Check sheet for the modelled part. Datum: model origin and axes. Units: mm. A direction names the side the tool comes from. Coordinates: 2 decimals unless noted, no trailing zeros. Loops run counter-clockwise (first coordinate to the right, second up) from the corner with the lowest first, then second, coordinate; pieces in that order, holes last. Notation, with made-up numbers: M 7,6.5 L 25,6.5 A26 cw 25,34.5 Z; hole C -23.5,62 d2. An arc over 180 degrees is marked long. Return JSON: item names as keys, results as strings.
from build123d import *

# Parameters (mm, degrees)
P_IDAT_VYSUNUT_M1_DEPTH  = 280
ODEBRAT_VYSUNUT_M1_DEPTH = 4
SKICA3_R                 = 4.15
ODEBRAT_VYSUNUT_M2_DEPTH = 4
ZKOSEN_1_SIZE            = 0.5
ZKOSEN_2_SIZE            = 0.5


with BuildPart() as part:
    # Skica1 → Přidat vysunutím1 (new body)
    with BuildSketch(Plane.XY):
        Polygon((0, 35), (0, 0), (35, 0), (35, 3), (3, 3), (3, 35), align=None)
    extrude(amount=P_IDAT_VYSUNUT_M1_DEPTH)

    # Skica2 → Odebrat vysunutím1 (cut)
    with BuildSketch(Plane.ZY):
        with BuildLine():
            Line((30, 21.65), (42, 21.65))
            ThreePointArc((42, 21.65), (46.15, 17.5), (42, 13.35))
            Line((42, 13.35), (30, 13.35))
            ThreePointArc((30, 13.35), (25.85, 17.5), (30, 21.65))
        make_face()
        with BuildLine():
            Line((238, 21.65), (250, 21.65))
            ThreePointArc((250, 21.65), (254.15, 17.5), (250, 13.35))
            Line((250, 13.35), (238, 13.35))
            ThreePointArc((238, 13.35), (233.85, 17.5), (238, 21.65))
        make_face()
    extrude(amount=-ODEBRAT_VYSUNUT_M1_DEPTH, mode=Mode.SUBTRACT)

    # Skica3 → Odebrat vysunutím2 (cut)
    with BuildSketch(Plane(origin=(0, 3, 0), x_dir=(-1, 0, 0), z_dir=(0, 1, 0))):
        with Locations((-22.5, 265)):
            Circle(SKICA3_R)
        with Locations((-22.5, 15)):
            Circle(SKICA3_R)
    extrude(amount=-ODEBRAT_VYSUNUT_M2_DEPTH, mode=Mode.SUBTRACT)

    # Zkosení1
    zkosen_1_edges = [part.edges().sort_by_distance(p)[0] for p in [
        (17.5, 0, 280),
        (3, 35, 140),
        (35, 3, 140),
        (35, 0, 140),
        (19, 3, 280),
        (3, 13.35, 36),
        (3, 19, 280),
        (3, 17.5, 46.15),
        (3, 21.65, 36),
        (3, 17.5, 25.85),
        (0, 17.5, 25.85),
        (0, 13.35, 36),
        (0, 17.5, 46.15),
        (0, 21.65, 36),
        (3, 13.35, 244),
        (3, 17.5, 254.15),
        (3, 21.65, 244),
        (3, 17.5, 233.85),
        (1.5, 35, 280),
        (0, 17.5, 233.85),
        (0, 13.35, 244),
        (0, 17.5, 254.15),
        (0, 21.65, 244),
        (3, 19, 0),
        (19, 3, 0),
        (0, 17.5, 280),
        (17.5, 0, 0),
        (0, 17.5, 0),
        (1.5, 35, 0),
    ]]
    chamfer(zkosen_1_edges, length=ZKOSEN_1_SIZE)

    # Zkosení2
    zkosen_2_edges = [part.edges().sort_by_distance(p)[0] for p in [
        (0, 35, 140),
    ]]
    chamfer(zkosen_2_edges, length=ZKOSEN_2_SIZE)


solid = part.part
1) Draft check along X on faces 4 (the face through (23.4, 1.52, 260.95)), 5 (the face through (2.64, 17.41, 233.71)), 6 (the face through (17, 0, 138)). Enter one of: +X half, -X half, draft (parallel to the pull), parting line (faces both ways), or undercut.
Answers:
{"face 4": "undercut", "face 5": "+X half", "face 6": "draft"}
2) Section check C-C on x = 22.5. Record the cut outline in (y, z).
Answers:
{"outline": "M 0,0.5 L 0.5,0 L 2.5,0 L 3,0.5 L 3,10.85 L 0,10.85 Z; M 0,19.15 L 3,19.15 L 3,260.85 L 0,260.85 Z; M 0,269.15 L 3,269.15 L 3,279.5 L 2.5,280 L 0.5,280 L 0,279.5 Z"}
3) Section check A-A on z = 15. Record the cut outline in (x, y).
Answers:
{"outline": "M 0,0 L 18.35,0 L 18.35,3 L 3,3 L 3,34.5 L 2.5,35 L 0.5,35 L 0,34.5 Z; M 26.65,0 L 34.5,0 L 35,0.5 L 35,2.5 L 34.5,3 L 26.65,3 Z"}
4) Go/stop test with flat-tipped pins: pin 1 Ø6.5 at (x, z) = (22.5, 15) entering from +Y; pin 2 Ø13.5 at (x, z) = (22.5, 265) entering from -Y; pin 3 Ø12 at (x, z) = (28, 140.5) entering from +Y; pin 4 Ø1.5 at (y, z) = (13, 246.5) entering from +X. Record where each tip stops, or that it passes through.
Answers:
{"pin 1": "through", "pin 2": "y = 0", "pin 3": "y = 3", "pin 4": "x = 3"}
5) Set-up check for faces 1 (the face through (19, 3, 138)), 2 (the face through (2.64, 17.59, 254.29)), 3 (the face through (0.365, 17.406, 25.716)): record each of +Z, -Z, +X, -X, +Y, -Y from which the full face is reachable in a straight line by a thin tool's end or side.
Answers:
{"face 1": "+Z, -Z, +X, +Y", "face 2": "+X", "face 3": "-X"}
6) Scan lines: line 1 along Z through (x, y) = (22, 1); line 2 along X through (y, z) = (1.4, 265); line 3 along Y through (x, z) = (15.5, 229.5). Record each from-to range of solid material in increasing order. Write a range as [from, to].
Answers:
{"line 1": "[0, 10.88], [19.12, 260.88], [269.12, 280]", "line 2": "[0, 18.35], [26.65, 35]", "line 3": "[0, 3]"}
7) Section check D-D on x = 11.5. Record the cut outline in (y, z).
Answers:
{"outline": "M 0,0.5 L 0.5,0 L 2.5,0 L 3,0.5 L 3,279.5 L 2.5,280 L 0.5,280 L 0,279.5 Z"}
8) Section check B-B on y = 17.5. Record the cut outline in (x, z).
Answers:
{"outline": "M 0,0.5 L 0.5,0 L 2.5,0 L 3,0.5 L 3,25.35 L 2.5,25.85 L 0.5,25.85 L 0,25.35 Z; M 0,46.65 L 0.5,46.15 L 2.5,46.15 L 3,46.65 L 3,233.35 L 2.5,233.85 L 0.5,233.85 L 0,233.35 Z; M 0,254.65 L 0.5,254.15 L 2.5,254.15 L 3,254.65 L 3,279.5 L 2.5,280 L 0.5,280 L 0,279.5 Z"}
